```python
from build123d import *

# Parameters (mm, degrees)
F0_W     = 5.1
F0_H     = 32.1
F1_DEPTH = 19.2
F3_DEPTH = 5.101


with BuildPart() as f1:
    # F0 (on Right) → F1 (new body)
    with BuildSketch(Plane.YZ):
        Rectangle(F0_W, F0_H)
        Polygon((2.55, -16.05), (-2.55, -16.05), (2.540138, -30.266205), (7.341638, -28.547019), align=None)
    extrude(amount=F1_DEPTH)

    # F2 (on face) → F3 (cut, through all)
    with BuildSketch(Plane(origin=(0, 2.55, 0), x_dir=(-1, 0, 0), z_dir=(0, 1, 0))):
        with BuildLine():
            ThreePointArc((-9.6, 2.75), (-12.004163, -3.054163), (-6.2, -0.65))
            ThreePointArc((-6.2, -0.65), (-7.195837, 1.754163), (-9.6, 2.75))
        make_face()
    extrude(amount=-F3_DEPTH, mode=Mode.SUBTRACT)


solid = f1.part
```
Source: CAD feature listing. Evaluate the final solid. Frame: model axes, mm. A direction names the side the tool comes from. Coordinates: 2 decimals unless noted, no trailing zeros. Write each loop counter-clockwise with the first axis right and the second up, starting at its lowest first coordinate (ties: lowest second). Pieces come first, ordered by that corner, then holes. Notation, with made-up numbers: (9.25, 22.25) - (54.25, 22.25) arc R17 cw to (54.25, 34.25) - close; hole circle Ø6 at (27, -3.5). An arc over 180 degrees is marked (long way). Answer as a JSON object with one key per item and string values.
Q1. First-contact query: pin 1 Ø1.5 at (x, z) = (14, -24) entering from -Y; pin 2 Ø9.5 at (x, z) = (7.5, 6) entering from +Y. Flat tips, straight axial feed; report the tip coordinate or a pass-through.
Ans:
{"pin 1": "stops at y = 0.03", "pin 2": "stops at y = 2.55"}
Q2. Section query C-C, the plane z = 9. Output: boundary loops of the cut face in (x, y).
Ans:
{"outline": "(0, -2.55) - (19.2, -2.55) - (19.2, 2.55) - (0, 2.55) - close"}
Q3. Section query D-D, the plane y = 1.25. Output: boundary loops of the cut face in (x, z), plus the area to 3 significant figures.
Ans:
{"outline": "(0, -26.66) - (19.2, -26.66) - (19.2, 16.05) - (0, 16.05) - close; hole circle Ø6.8 at (9.6, -0.65)", "area": "784 mm2"}
Q4. Section query B-B, the plane x = 16. Output: boundary loops of the cut face in (y, z), plus the area to 3 significant figures.
Ans:
{"outline": "(-2.55, -16.05) - (2.54, -30.27) - (7.34, -28.55) - (2.55, -16.05) - (2.55, 16.05) - (-2.55, 16.05) - close", "area": "234 mm2"}
Q5. Set-up query: faces 1 (the flat face through (0, 1, -7)), 2 (the flat face through (9, 2.55, 3)). Return all of +Z, -Z, +X, -X, +Y, -Y with unobstructed straight access to the full face (end or side cutting, diameter ignored); none if empty.
Ans:
{"face 1": "+Z, -Z, -X, +Y, -Y", "face 2": "+Z, +X, -X, +Y"}
Q6. Material intervals for line 1 (X direction, y = -1.25, z = -0.65); line 2 (Y direction, x = 7, z = 3); line 3 (Y direction, x = 9.5, z = -19.5), sorted ascending. Write a range as [from, to].
Ans:
{"line 1": "x = [0, 6.2], [13, 19.2]", "line 2": "y = [-2.55, 2.55]", "line 3": "y = [-1.31, 3.87]"}
Q7. Section query A-A, the plane y = -2. Output: boundary loops of the cut face in (x, z).
Ans:
{"outline": "(0, -17.59) - (19.2, -17.59) - (19.2, 16.05) - (0, 16.05) - close; hole circle Ø6.8 at (9.6, -0.65)"}
